```python
from build123d import *

# Parameters (mm, degrees)
SKETCH_1_R          = 12.5
EXTRUDE_1_DEPTH     = 35
SKETCH_2_R          = 3.5
EXTRUDE_2_DEPTH     = 2.5
SKETCH_3_R          = 2
EXTRUDE_3_DEPTH     = 10
CUT_EXTRUDE_START   = -10
CUT_EXTRUDE_1_DEPTH = 10
SKETCH_5_R          = 1.5
CUT_EXTRUDE_2_DEPTH = 4.5


with BuildPart() as part:
    # 草图1 → 凸台-拉伸1 (new body)
    with BuildSketch(Plane.XY):
        Circle(SKETCH_1_R)
    extrude(amount=EXTRUDE_1_DEPTH)

    # 草图2 → 凸台-拉伸2 (add)
    with BuildSketch(Plane.XY.offset(35)):
        Circle(SKETCH_2_R)
    extrude(amount=EXTRUDE_2_DEPTH)

    # 草图3 → 凸台-拉伸3 (add)
    with BuildSketch(Plane.XY.offset(37.5)):
        Circle(SKETCH_3_R)
    extrude(amount=EXTRUDE_3_DEPTH)

    # 草图4 → 切除-拉伸1 (cut)
    with BuildSketch(Plane.XY.offset(47.5).offset(CUT_EXTRUDE_START)):
        with BuildLine():
            Line((-1.5, 1.322875656), (-1.5, -1.322875656))
            ThreePointArc((-1.5, -1.322875656), (-2, 0), (-1.5, 1.322875656))
        make_face()
    extrude(amount=CUT_EXTRUDE_1_DEPTH, mode=Mode.SUBTRACT)

    # 草图5 → 切除-拉伸2 (cut)
    with BuildSketch(Plane.XY.offset(35)):
        with Locations((0, 8.5)):
            Circle(SKETCH_5_R)
        with Locations((0, -8.5)):
            Circle(SKETCH_5_R)
    extrude(amount=-CUT_EXTRUDE_2_DEPTH, mode=Mode.SUBTRACT)


solid = part.part
```
Input: part model. Units: mm. Frame: model coordinates. A direction names the side the tool comes from. Give positions to 0.01 mm unless a question says otherwise; leave off trailing zeros. Order: outer loops, then holes, each group sorted by start corner. A loop starts at its lowest first (then second) coordinate and runs counter-clockwise, first axis right, second up. Notation, with made-up numbers: M -36,80.5 L -19,80.5 A14 ccw -19,86.5 Z; hole C 28,3 d10. An arc over 180 degrees is marked long. Return JSON: item names as keys, results as strings.
1) Mould query, pull axis X, two halves, no side actions, for faces 1 (the face through (0, 0, 47.5)), 2 (the face through (0, -8, 30.5)), 3 (the face through (2, 0, 42)). Classes: released by +X, released by -X, zero draft, split by the parting line, or undercut.
Taken from the geometry:
{"face 1": "zero draft", "face 2": "undercut", "face 3": "split by the parting line"}
2) Contact query for flat-ended pins moving along their axis: pin 1 (4 mm diameter, centred on y = -9.5, z = 10, fed in from +X); pin 2 (10 mm diameter, centred on x = 5.5, z = 17.5, fed in from -Y); pin 3 (2.5 mm diameter, centred on x = -0.5, y = 9, fed in from +Z). Output: stop coordinate, or through.
Taken from the geometry:
{"pin 1": "stops at x = 10", "pin 2": "stops at y = -12.49", "pin 3": "stops at z = 35"}
3) Access query for faces 4 (the face through (-2, 0, 37.5)), 5 (the face through (0, 0, 0)), 6 (the face through (-1.5, 0, 42)). Directions: +Z, -Z, +X, -X, +Y, -Y. A direction counts if a zero-diameter tool reaches every point of the face in a straight line with its end or side. Return the directions, or none.
Taken from the geometry:
{"face 4": "+Z", "face 5": "-Z, +X, -X, +Y, -Y", "face 6": "+Z, -X, +Y, -Y"}
4) Section query B-B on y = 0. Output: boundary loops of the cut face in (x, z).
Taken from the geometry:
{"outline": "M -12.5,0 L 12.5,0 L 12.5,35 L 3.5,35 L 3.5,37.5 L 2,37.5 L 2,47.5 L -1.5,47.5 L -1.5,37.5 L -3.5,37.5 L -3.5,35 L -12.5,35 Z"}
5) Section query D-D on y = -8.5. Output: boundary loops of the cut face in (x, z), and give its area (3 significant figures).
Taken from the geometry:
{"outline": "M -9.17,0 L 9.17,0 L 9.17,35 L 1.5,35 L 1.5,30.5 L -1.5,30.5 L -1.5,35 L -9.17,35 Z", "area": "628 mm2"}
6) Section query A-A on x = 0. Output: boundary loops of the cut face in (y, z), and give its area (4 significant figures).
Taken from the geometry:
{"outline": "M -12.5,0 L 12.5,0 L 12.5,35 L 10,35 L 10,30.5 L 7,30.5 L 7,35 L 3.5,35 L 3.5,37.5 L 2,37.5 L 2,47.5 L -2,47.5 L -2,37.5 L -3.5,37.5 L -3.5,35 L -7,35 L -7,30.5 L -10,30.5 L -10,35 L -12.5,35 Z", "area": "905.5 mm2"}
7) Section query C-C on z = 27.5. Output: boundary loops of the cut face in (x, y).
Taken from the geometry:
{"outline": "C 0,0 d25"}
8) Line query: L1, parallel to Y at x = 0, z = 32; L2, parallel to Z at x = 7.75, y = 6.75; L3, parallel to Y at x = 0.5, z = 15.5. Output: solid intervals per line, ascending. Write a range as [from, to].
Taken from the geometry:
{"L1": "y = [-12.5, -10], [-7, 7], [10, 12.5]", "L2": "z = [0, 35]", "L3": "y = [-12.49, 12.49]"}
